The model under review builds one solid part; all positions refer to its coordinate system, in mm. A direction names the side the tool comes from. Give positions to 0.01 mm unless a question says otherwise; leave off trailing zeros. Loops run counter-clockwise (first coordinate to the right, second up) from the corner with the lowest first, then second, coordinate; pieces in that order, holes last. Notation, with made-up numbers: (62, -3) -> (111, -3) arc R27 cw to (111, 32) -> close; hole circle Ø10 at (-38, -24). An arc over 180 degrees is marked (long way). Write each question's results on one line, items separated by ' | '. Start each with the question number.
Q1. Machinability: for faces 1 (the face through (1.08, 4.88, 4.56)), 2 (the face through (1.73, 7.81, 12.29)), 3 (the face through (2.17, 9.76, 8.71)), which of the approach directions +Z, -Z, +X, -X, +Y, -Y give a long, thin tool a straight path to every point of the face, cutting with its end or side? Answer none if there is none.
Q2. We need section C-C (z = 8). Write out the cut boundary in (x, y).
Q3. We need section D-D (z = 14). Write out the cut boundary in (x, y), plus the area to 3 significant figures.
Q4. Wall thickness on L1, parallel to Y at x = 0, z = 6.5; L2, parallel to Z at x = 1, y = -12: over which ranges is each line inside the solid? List them lowest first. Write a range as [from, to].
Q5. Insertion check: pin 1 Ø1.5 at (y, z) = (-9.5, 3) entering from -X; pin 2 Ø12 at (x, y) = (-1.5, 0) entering from +Z; pin 3 Ø8 at (x, z) = (-10.5, 7.5) entering from +Y; pin 4 Ø6 at (x, z) = (-2, 8.5) entering from +Y. Each pin has a flat end and moves straight along its axis. Give the tip position at first contact, or say it passes through.
Q6. Mouldability with a two-part tool opening along Y and no side actions: class faces 4 (the face through (2, 5, 9)), 5 (the face through (12.637, 9.69, 13.486)), 6 (the face through (7, 7, 15)) as released by +Y, released by -Y, zero draft, split by the parting line, or undercut.
from build123d import *

# Parameters (mm, degrees)
F2_SIZE = 0.5
F3_SIZE = 0.5


with BuildPart() as f1:
    # F0 (on Front) → F1 (revolve)
    with BuildSketch(Plane.XZ):
        with BuildLine():
            Line((-15.92432, 12), (-10, 12))
            Line((-10, 12), (-10, 6))
            Line((-10, 6), (-8, 6))
            Line((-8, 6), (-8, 0))
            Line((-8, 0), (-5, 0))
            Line((-5, 0), (-5, 9))
            Line((-5, 9), (-7.5, 9))
            ThreePointArc((-7.5, 9), (-7.853553, 9.146447), (-8, 9.5))
            Line((-8, 9.5), (-8, 15))
            Line((-8, 15), (-15.92432, 15))
            Line((-15.92432, 15), (-15.92432, 12))
        make_face()
    revolve(axis=Axis((0, 0, 8.069702), (0, 0, 1)))

    # F2
    f2_edges = [f1.edges().sort_by_distance(p)[0] for p in [
        (8, 0, 6),
    ]]
    chamfer(f2_edges, length=F2_SIZE)

    # F3
    f3_edges = [f1.edges().sort_by_distance(p)[0] for p in [
        (15.92432, 0, 12),
        (15.92432, 0, 15),
        (10, 0, 12),
    ]]
    chamfer(f3_edges, length=F3_SIZE)


solid = f1.part
Output:
1) face 1: +Z, -Z | face 2: +Z | face 3: -Z
2) outline: circle Ø20 at (0, 0); hole circle Ø10 at (0, 0)
3) outline: circle Ø31.85 at (0, 0); hole circle Ø16 at (0, 0) | area: 596 mm2
4) L1: [-10, -5], [5, 10] | L2: [12, 15]
5) pin 1: through | pin 2: z = 9 | pin 3: y = 7.6 | pin 4: y = 10
6) face 4: undercut | face 5: split by the parting line | face 6: zero draft
